from build123d import *

# Parameters (mm, degrees)
SKETCH_W    = 40
SKETCH_H    = 40
SKETCH_W_2  = 36
SKETCH_H_2  = 36
PAD_DEPTH   = 613
SKETCH001_R = 3.3
HOLE_DEPTH  = 40.001


with BuildPart() as part:
    # Sketch → Pad (new body)
    with BuildSketch(Plane.XZ):
        Rectangle(SKETCH_W, SKETCH_H)
        Rectangle(SKETCH_W_2, SKETCH_H_2, mode=Mode.SUBTRACT)
    extrude(amount=PAD_DEPTH)

    # Sketch001 → Hole (cut, through all)
    with BuildSketch(Plane(origin=(20, 0, 0), x_dir=(0, 0, 1), z_dir=(1, 0, 0))):
        with Locations((0, 25)):
            Circle(SKETCH001_R)
        with Locations((0, 50)):
            Circle(SKETCH001_R)
        with Locations((0, 588)):
            Circle(SKETCH001_R)
        with Locations((0, 563)):
            Circle(SKETCH001_R)
    extrude(amount=-HOLE_DEPTH, mode=Mode.SUBTRACT)


solid = part.part
Design review of the part built by this model. Coordinates are the model's own, in mm. A direction names the side the tool comes from. Round coordinates to 2 decimals unless told otherwise and drop trailing zeros. Write each loop counter-clockwise with the first axis right and the second up, starting at its lowest first coordinate (ties: lowest second). Pieces come first, ordered by that corner, then holes. Notation, with made-up numbers: (6, 23.25) - (29, 23.25) arc R22 ccw to (29, 56.25) - close; hole circle Ø2 at (28, -2.5). An arc over 180 degrees is marked (long way). Use a Markdown table: item, result. Add a question column.
1. We need section C-C (z = 12). State the section outline as (x, y) points.
2. We need section B-B (y = -407). State the section outline as (x, z) points.
3. We need section A-A (x = -6). State the section outline as (y, z) points.
4. Wall thickness on probe 1 along Z at (x, y) = (-17, -479); probe 2 along Z at (x, y) = (19, -25): over which ranges is each line inside the solid? List them lowest first.
5. Mouldability with a two-part tool opening along Z and no side actions: class faces 1 (the face through (0, -302, -20)), 2 (the face through (-18, -302, 0)), 3 (the face through (0, -302, 20)), 4 (the face through (-2, -613, -19)) as +Z half, -Z half, draft (parallel to the pull), parting line (faces both ways), or undercut.
6. For faces 5 (the face through (18, -302, 0)), 6 (the face through (-2, 0, -19)), list the 3-axis set-ups (+Z, -Z, +X, -X, +Y, -Y) from which the entire face can be reached by the end or side of a thin tool; tool diameter is ignored.
Output:
| question | item | result |
|---|---|---|
| 1 | outline | (-20, -613) - (-18, -613) - (-18, 0) - (-20, 0) - close; (18, -613) - (20, -613) - (20, 0) - (18, 0) - close |
| 2 | outline | (-20, -20) - (20, -20) - (20, 20) - (-20, 20) - close; hole (-18, -18) - (18, -18) - (18, 18) - (-18, 18) - close |
| 3 | outline | (-613, -20) - (0, -20) - (0, -18) - (-613, -18) - close; (-613, 18) - (0, 18) - (0, 20) - (-613, 20) - close |
| 4 | probe 1 | z = -20 to -18, 18 to 20 |
| 4 | probe 2 | z = -20 to -3.3, 3.3 to 20 |
| 5 | face 1 | -Z half |
| 5 | face 2 | undercut |
| 5 | face 3 | +Z half |
| 5 | face 4 | draft |
| 6 | face 5 | +Y, -Y |
| 6 | face 6 | +Z, -Z, +X, -X, +Y |
